Can you work these out from the model? Positions are in its coordinate system, mm. Face numbers are marked on the shaded views. A direction names the side the tool comes from. Coordinates: 2 decimals unless noted, no trailing zeros. Loops run counter-clockwise (first coordinate to the right, second up) from the corner with the lowest first, then second, coordinate; pieces in that order, holes last. Notation, with made-up numbers: (56, -29) - (101, -29) arc R16 ccw to (101, -8) - close; hole circle Ø11 at (18, -37). An arc over 180 degrees is marked (long way). Put each result on its own line as item: value. Start each with the question number.
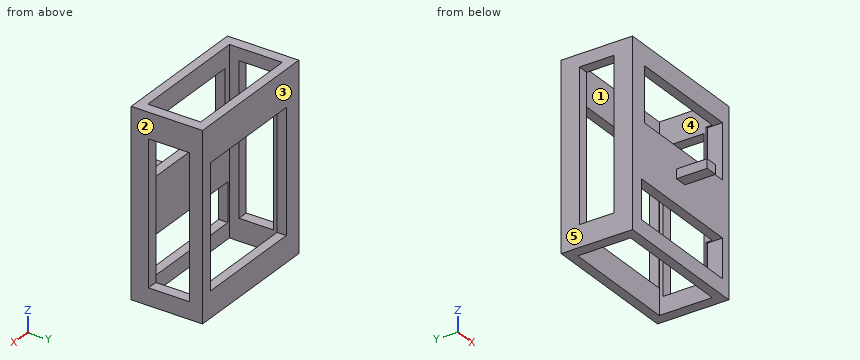
from build123d import *

# Parameters (mm, degrees)
F1_DEPTH  = 30
F2_W      = 6.674083
F2_H      = 23.102594
F3_DEPTH  = 2.5
F4_W      = 5.588458
F4_H      = 24.429547
F5_DEPTH  = 2.5
F6_W      = 18.183109
F6_H      = 19.870534
F7_DEPTH  = 2.5
F8_W      = 19.441772
F8_H      = 6.327746
F8_W_2    = 18.70812
F8_H_2    = 8.895528
F9_DEPTH  = 2.5
F10_W     = 2
F10_H     = 1.5
F11_DEPTH = 5


with BuildPart() as f1:
    # F0 (on Top) → F1 (new body)
    with BuildSketch(Plane.XY):
        Polygon((-5.624948, 38.338026), (-16.317087, 38.338026), (-16.317087, 26.738026), (-3.303813, 26.738026), (-3.164812, 26.738026), (6.682913, 26.738026), (6.682913, 38.338026), (-5.508062, 38.338026), align=None)
        Polygon((-14.575047, 32.538026), (-14.575047, 36.838026), (-5.625147, 36.838026), (-5.508261, 36.838026), (4.924953, 36.838026), (4.924953, 28.238026), (-3.164812, 28.238026), (-3.303813, 28.238026), (-14.575047, 28.238026), (-14.575047, 32.102089), align=None, mode=Mode.SUBTRACT)
    extrude(amount=F1_DEPTH)

    # F2 (on face) → F3 (cut)
    with BuildSketch(Plane.YZ.offset(6.682913)):
        with Locations((32.882399, 14.318564)):
            Rectangle(F2_W, F2_H)
    extrude(amount=-F3_DEPTH, mode=Mode.SUBTRACT)

    # F4 (on face) → F5 (cut)
    with BuildSketch(Plane(origin=(-16.317087, 0, 0), x_dir=(0, -1, 0), z_dir=(-1, 0, 0))):
        with Locations((-32.585687, 15.768258)):
            Rectangle(F4_W, F4_H)
    extrude(amount=-F5_DEPTH, mode=Mode.SUBTRACT)

    # F6 (on face) → F7 (cut)
    with BuildSketch(Plane(origin=(0, 38.338026, 0), x_dir=(-1, 0, 0), z_dir=(0, 1, 0))):
        with Locations((4.255847, 14.15753)):
            Rectangle(F6_W, F6_H)
    extrude(amount=-F7_DEPTH, mode=Mode.SUBTRACT)

    # F8 (on face) → F9 (cut)
    with BuildSketch(Plane.XZ.offset(-26.738026)):
        with Locations((-4.50602, 5.721706)):
            Rectangle(F8_W, F8_H)
        with Locations((-4.139194, 22.320578)):
            Rectangle(F8_W_2, F8_H_2)
    extrude(amount=-F9_DEPTH, mode=Mode.SUBTRACT)

    # F10 (on face) → F11 (join)
    with BuildSketch(Plane.XZ.offset(-26.738026)):
        with Locations((-4.817087, 13.603965)):
            Rectangle(F10_W, F10_H)
    extrude(amount=F11_DEPTH)


solid = f1.part
Q1. We'd pull the mould along Y, two halves only. Please class the marked faces 3, 4 and 5: released by +Y, released by -Y, zero draft, split by the parting line, or undercut.
Q2. I want a section at D-D on z = 6. List the corners of the cut face in (x, y) for me, and give its area (3 significant figures).
Q3. I want a section at B-B on z = 10. List the corners of the cut face in (x, y) for me.
Q4. On a 3-axis mill with a long thin cutter (end or side, diameter ignored), from which of +Z, -Z, +X, -X, +Y, -Y can I reach the whole of each face in a straight line? I mean the marked faces 1 and 2. Say none if no direction works.
Q5. I want a section at A-A on y = 32.5. List the corners of the cut face in (x, z) for me.
Q6. I want a section at C-C on x = -13. List the corners of the cut face in (y, z) for me, and give its area (3 significant figures).
Q7. Will these pins go through, and if not, where does the flat tip stop? pin 1 (1.9 mm diameter, centred on x = 6, y = 33, fed in from -Z); pin 2 (6 mm diameter, centred on x = -11, y = 31.5, fed in from +Z); pin 3 (1.2 mm diameter, centred on y = 24, z = 13.5, fed in from +X); pin 4 (5 mm diameter, centred on x = -10.5, z = 11, fed in from +Y).
Q8. Please list where these lines run through material, in increasing order: line 1 along Z through (x, y) = (-2, 27); line 2 along Y through (x, z) = (-15, 4.25); line 3 along Y through (x, z) = (-2.25, 27.5). Write a range as [from, to].
Calculated:
1. face 3: released by +Y
1. face 4: undercut
1. face 5: zero draft
2. outline: (-16.32, 26.74) - (-14.23, 26.74) - (-14.23, 28.24) - (-14.58, 28.24) - (-14.58, 29.79) - (-16.32, 29.79) - close; (-16.32, 35.38) - (-14.58, 35.38) - (-14.58, 36.84) - (-13.35, 36.84) - (-13.35, 38.34) - (-16.32, 38.34) - close; (4.84, 36.84) - (4.92, 36.84) - (4.92, 36.22) - (6.68, 36.22) - (6.68, 38.34) - (4.84, 38.34) - close; (4.92, 29.24) - (5.21, 29.24) - (5.21, 26.74) - (6.68, 26.74) - (6.68, 29.55) - (4.92, 29.55) - close
2. area: 20.9 mm2
3. outline: (-16.32, 26.74) - (6.68, 26.74) - (6.68, 29.55) - (4.92, 29.55) - (4.92, 28.24) - (-14.58, 28.24) - (-14.58, 29.79) - (-16.32, 29.79) - close; (-16.32, 35.38) - (-14.58, 35.38) - (-14.58, 36.84) - (-13.35, 36.84) - (-13.35, 38.34) - (-16.32, 38.34) - close; (4.84, 36.84) - (4.92, 36.84) - (4.92, 36.22) - (6.68, 36.22) - (6.68, 38.34) - (4.84, 38.34) - close
4. face 1: +Z, -Z
4. face 2: +Z, -Z, +X, +Y, -Y
5. outline: (-16.32, 0) - (-14.58, 0) - (-14.58, 3.55) - (-16.32, 3.55) - close; (-16.32, 27.98) - (-14.58, 27.98) - (-14.58, 30) - (-16.32, 30) - close; (4.92, 0) - (6.68, 0) - (6.68, 2.77) - (4.92, 2.77) - close; (4.92, 25.87) - (6.68, 25.87) - (6.68, 30) - (4.92, 30) - close
6. outline: (26.74, 0) - (28.24, 0) - (28.24, 2.56) - (26.74, 2.56) - close; (26.74, 8.89) - (28.24, 8.89) - (28.24, 17.87) - (26.74, 17.87) - close; (26.74, 26.77) - (28.24, 26.77) - (28.24, 30) - (26.74, 30) - close; (36.84, 0) - (38.34, 0) - (38.34, 4.22) - (36.84, 4.22) - close; (36.84, 24.09) - (38.34, 24.09) - (38.34, 30) - (36.84, 30) - close
6. area: 37.4 mm2
7. pin 1: z = 0
7. pin 2: through
7. pin 3: x = -3.82
7. pin 4: y = 28.24
8. line 1: [0, 2.56], [8.89, 17.87], [26.77, 30]
8. line 2: [26.74, 29.79], [35.38, 38.34]
8. line 3: [26.74, 28.24], [36.84, 38.34]
